```python
from build123d import *

# Parameters (mm, degrees)
BOSS_EXTRU_1_DEPTH      = 5
ESQUISSE2_R             = 9
ENL_V_MAT_EXTRU_1_DEPTH = 170.03549923


with BuildPart() as part:
    # Esquisse1 → Boss.-Extru.1 (new body)
    with BuildSketch(Plane.XY):
        Polygon((29.5, 154), (29.5, 157), (33, 157), (33, 162), (38, 162), (38, 157), (48, 157), (15, 0), (10, 0), (10, -5), (5, -5), (5, 0), (1.5, 0), (1.5, 3), (2.6, 3), (2.6, 5.3), (1.5, 5.3), (1.5, 10), (-1.5, 10), (-1.5, 5.3), (-2.6, 5.3), (-2.6, 3), (-1.5, 3), (-1.5, 0), (-5, 0), (-5, -5), (-10, -5), (-10, 0), (-20, 0), (13, 157), (18, 157), (18, 162), (23, 162), (23, 157), (26.5, 157), (26.5, 154), (25.4, 154), (25.4, 151.7), (26.5, 151.7), (26.5, 147), (29.5, 147), (29.5, 151.7), (30.6, 151.7), (30.6, 154), align=None)
    extrude(amount=BOSS_EXTRU_1_DEPTH)

    # Esquisse2 → Enlèv. mat.-Extru.1 (cut, through all)
    with BuildSketch(Plane.XY.offset(5)):
        with Locations((24.411695113, 129.442936805)):
            Circle(ESQUISSE2_R)
        with Locations((18.404488272, 100.050531902)):
            Circle(ESQUISSE2_R)
        with Locations((12.397281431, 70.658126999)):
            Circle(ESQUISSE2_R)
        with Locations((6.390074589, 41.265722097)):
            Circle(ESQUISSE2_R)
    extrude(amount=-ENL_V_MAT_EXTRU_1_DEPTH, mode=Mode.SUBTRACT)


solid = part.part
```
Check sheet for the modelled part. Datum: model origin and axes. Units: mm. A direction names the side the tool comes from. Round coordinates to 2 decimals unless told otherwise and drop trailing zeros. Loops run counter-clockwise (first coordinate to the right, second up) from the corner with the lowest first, then second, coordinate; pieces in that order, holes last. Notation, with made-up numbers: (78, -13.5) - (130, -13.5) arc R28 ccw to (130, 11.5) - close; hole circle Ø4 at (28, 28). An arc over 180 degrees is marked (long way). Answer as a JSON object with one key per item and string values. Group by question number.
Q1. Scan lines: line 1 along X through (y, z) = (7, 1.55); line 2 along X through (y, z) = (77, 4.25); line 3 along X through (y, z) = (32, 1.8). Record each from-to range of solid material in increasing order. Write a range as [from, to].
Q2. Sectioned sample at A-A, the plane y = 34.5. Enter the section's corners in (x, z) (3 decimals), plus the area to 3 significant figures.
Q3. Sectioned sample at C-C, the plane z = 2.3. Count the separate pieces of the cut face and the enclosed holes in it, plus the area to 3 significant figures.
Q4. Mould release check, pull along Y, two halves, no side actions. Record for faces 4 (the face through (23, 160, 2)), 5 (the face through (25, 157, 2)), 6 (the face through (10.45, 61.87, 2.54)): released by +Y, released by -Y, zero draft, split by the parting line, or undercut.
Q5. Gauge pin test, flat ends, axial feed: P1, Ø1.8, axis at x = 31, z = 3.5, coming from the +Y side; P2, Ø2.5, axis at y = -1.5, z = 3, coming from the -X side; P3, Ø1.5, axis at y = -2.5, z = 3.5, coming from the +X side; P4, Ø4, axis at x = 4.5, y = 118.5, coming from the +Z side. Record the tip position at first contact, or that the pin passes through.
Q6. Set-up check for faces 1 (the face through (33, 159, 2)), 2 (the face through (10, -2, 2)), 3 (the face through (-1.5, 8, 2)): record each of +Z, -Z, +X, -X, +Y, -Y from which the full face is reachable in a straight line by a thin tool's end or side.
Q7. Sectioned sample at B-B, the plane x = 11.5. Enter the section's corners in (y, z), plus the area to 3 significant figures.
Q8. Sectioned sample at D-D, the plane y = 113. Enter the section's corners in (x, z).
Solution:
{
 "1": {"line 1": "x = [-18.53, -1.5], [1.5, 16.47]", "line 2": "x = [-3.82, 6.01], [18.78, 31.18]", "line 3": "x = [-13.27, 21.73]"},
 "2": {"outline": "(-12.748, 0) - (0.455, 0) - (0.455, 5) - (-12.748, 5) - close; (12.325, 0) - (22.252, 0) - (22.252, 5) - (12.325, 5) - close", "area": "116 mm²"},
 "3": {"separate pieces": "1", "enclosed holes": "4", "area": "4,510 mm²"},
 "4": {"face 4": "zero draft", "face 5": "released by +Y", "face 6": "undercut"},
 "5": {"P1": "stops at y = 157", "P2": "stops at x = -10", "P3": "stops at x = 10", "P4": "stops at z = 5"},
 "6": {"face 1": "+Z, -Z, +Y", "face 2": "+Z, -Z, +X, -Y", "face 3": "+Z, -Z, -Y"},
 "7": {"outline": "(0, 0) - (33.86, 0) - (33.86, 5) - (0, 5) - close; (48.67, 0) - (61.7, 0) - (61.7, 5) - (48.67, 5) - close; (79.61, 0) - (94.28, 0) - (94.28, 5) - (79.61, 5) - close; (105.82, 0) - (149.86, 0) - (149.86, 5) - (105.82, 5) - close", "area": "528 mm²"},
 "8": {"outline": "(3.75, 0) - (38.75, 0) - (38.75, 5) - (3.75, 5) - close"}
}
